The listing builds one solid part. Answer for the finished solid, in the listing's coordinates (mm). A direction names the side the tool comes from. Give positions to 0.01 mm unless a question says otherwise; leave off trailing zeros. Write each loop counter-clockwise with the first axis right and the second up, starting at its lowest first coordinate (ties: lowest second). Pieces come first, ordered by that corner, then holes.
```python
from build123d import *

# Parameters (mm, degrees)
SKETCH1_W           = 6.9
SKETCH1_H           = 6.9
BOSS_EXTRUDE1_DEPTH = 7.5
FILLET2_R           = 3.5
FILLET3_R           = 3.5
FILLET4_R           = 3.5
FILLET5_DEPTH       = 7.5
SKETCH2_R           = 3.429778851
BOSS_EXTRUDE3_DEPTH = 7.5
SKETCH4_W           = 6.879778851
SKETCH4_H           = 1.06
CUT_EXTRUDE6_DEPTH  = 15
CUT_EXTRUDE8_DEPTH  = 15


with BuildPart() as part:
    # Sketch1 → Boss-Extrude1 (new body)
    with BuildSketch(Plane.XY):
        with Locations((3.45, 3.45)):
            Rectangle(SKETCH1_W, SKETCH1_H)
        Polygon((3.45, 5.9), (4.4, 5.9), (4.4, 4.4), (5.9, 4.4), (5.9, 2.5), (4.4, 2.5), (4.4, 1), (2.5, 1), (2.5, 2.5), (1, 2.5), (1, 4.4), (2.5, 4.4), (2.5, 5.9), align=None, mode=Mode.SUBTRACT)
    extrude(amount=BOSS_EXTRUDE1_DEPTH)

    # Fillet2
    fillet2_edges = [part.edges().sort_by_distance(p)[0] for p in [
        (0, 6.9, 3.75),
    ]]
    fillet(fillet2_edges, radius=FILLET2_R)

    # Fillet3
    # the kernel refuses this fillet: 3.5 mm, written as the material it takes off along each edge
    with BuildSketch(Plane(origin=(6.9, 6.9, -8.746427842), x_dir=(-1, 0, 0), z_dir=(0, 0, 1))) as fillet3_piece_1:
        with BuildLine():
            CenterArc((3.5, 3.498571137), FILLET3_R, 180, 88.362754922)
            Line((0, 3.498571137), (-0.07, 3.498571137))
            Line((-0.07, 3.498571137), (-0.07, 0))
            Line((-0.07, 0), (0, -0.07))
            ThreePointArc((0, -0.07), (1.7, -0.07), (3.398, -0.069971423))
            Line((3.398, -0.069971423), (3.4, 0))
        make_face()
    extrude(amount=24.992855685, mode=Mode.SUBTRACT)

    # Fillet4
    # the kernel refuses this fillet: 3.5 mm, written as the material it takes off along each edge
    with BuildSketch(Plane(origin=(6.9, 0, -8.746529216), x_dir=(0, 1, 0), z_dir=(0, 0, 1))) as fillet4_piece_1:
        with BuildLine():
            CenterArc((3.5, 3.498611686), FILLET4_R, 180, 88.386155146)
            Line((0, 3.498611686), (-0.07, 3.498611686))
            Line((-0.07, 3.498611686), (-0.07, 0))
            Line((-0.07, 0), (0, -0.07))
            ThreePointArc((0, -0.07), (1.700714432, -0.07), (3.39945744, -0.069972234))
            Line((3.39945744, -0.069972234), (3.401428863, 0))
        make_face()
    extrude(amount=24.993058431, mode=Mode.SUBTRACT)

    # Fillet5: read off the stored shape, not the designer's step
    # Fillet5 outline → Fillet5 (cut)
    with BuildSketch(Plane.XY):
        with BuildLine():
            Line((0, 0), (3.401388314, 0))
            ThreePointArc((3.401388314, 0), (1.007751346, 1.041234576), (0.000347304, 3.449305272))
            ThreePointArc((0.000347304, 3.449305272), (8.6827e-05, 3.424653248), (0, 3.4))
            Line((0, 3.4), (0, 0))
        make_face()
    extrude(amount=FILLET5_DEPTH, mode=Mode.SUBTRACT)

    # Sketch2 → Boss-Extrude3 (add)
    with BuildSketch(Plane.XY):
        with Locations((3.45, 3.449305272)):
            Circle(SKETCH2_R)
        with BuildLine():
            Line((5.5103837, 5.418396181), (1.3896163, 5.418396181))
            ThreePointArc((1.3896163, 5.418396181), (0.6, 3.449305272), (1.3896163, 1.480214363))
            Line((1.3896163, 1.480214363), (5.5103837, 1.480214363))
            ThreePointArc((5.5103837, 1.480214363), (6.3, 3.449305272), (5.5103837, 5.418396181))
        make_face(mode=Mode.SUBTRACT)
    extrude(amount=-BOSS_EXTRUDE3_DEPTH)

    # Sketch4 → Cut-Extrude6 (cut)
    with BuildSketch(Plane(origin=(0, 0, -7.5), x_dir=(-1, 0, 0), z_dir=(0, 0, -1))):
        with Locations((-3.439889426, 0.53)):
            Rectangle(SKETCH4_W, SKETCH4_H)
    extrude(amount=-CUT_EXTRUDE6_DEPTH, mode=Mode.SUBTRACT)

    # Sketch6 → Cut-Extrude8 (cut)
    with BuildSketch(Plane(origin=(0, 0, -7.5), x_dir=(-1, 0, 0), z_dir=(0, 0, -1))):
        Polygon((-3.455260778, 6.975766387), (-6.044608069, 6.975766387), (-6.044608069, 5.876947105), (-3.455260778, 5.876947105), (-1.008353024, 5.876947105), (-1.008353024, 6.975766387), align=None)
    extrude(amount=-CUT_EXTRUDE8_DEPTH, mode=Mode.SUBTRACT)


solid = part.part
```
Item 1: Each of these flat-tipped pins is pushed along its axis until it touches: P1, Ø0.7, axis at y = 2, z = 4.5, coming from the +X side; P2, Ø1.5, axis at x = 5, y = 4.5, coming from the -Z side; P3, Ø1.2, axis at y = 5.5, z = 3, coming from the +X side. Where does it stop, or does it pass through?
Conclusion:
P1: stops at x = 6.71
P2: stops at z = 0
P3: stops at x = 6.56
Item 2: Which of the six approach directions +Z, -Z, +X, -X, +Y, -Y give full straight-line access (tool end or side, diameter ignored) to faces 4 (the face through (2.5, 5, 4)), 5 (the face through (6.3, 3.4, -3.7)), 6 (the face through (6.88, 3.44, -3.7)), 7 (the face through (0.27, 4.75, 3.8)), 8 (the face through (3.4, 5.6, -7.5))?
Conclusion:
face 4: +Z, +Y, -Y
face 5: -Z
face 6: -Z, +X
face 7: +Z, -Z, -X, +Y
face 8: -Z, +X, -X, +Y, -Y
Item 3: A cutting plane is placed at B-B, the plane x = 2.25. Give the vertices of the cut face in (y, z).
Conclusion:
outline: (1.06, -7.5) - (1.48, -7.5) - (1.48, 0) - (2.5, 0) - (2.5, 7.5) - (1.06, 7.5) - close; (4.4, 0) - (5.42, 0) - (5.42, -7.5) - (5.88, -7.5) - (5.88, 7.5) - (4.4, 7.5) - close
Item 4: A cutting plane is placed at A-A, the plane z = 3. Give the vertices of the cut face in (x, y).
Conclusion:
outline: (0, 3.45) arc R3.5 ccw to (0.99, 1.06) - (2.5, 1.06) - (2.5, 2.5) - (1, 2.5) - (1, 4.4) - (2.5, 4.4) - (2.5, 5.88) - (1.03, 5.88) arc R3.5 ccw to start; (4.4, 1.06) - (5.91, 1.06) arc R3.5 ccw to (6.9, 3.4) arc R3.5 ccw to (5.87, 5.88) - (4.4, 5.88) - (4.4, 4.4) - (5.9, 4.4) - (5.9, 2.5) - (4.4, 2.5) - close
Item 5: Determine the mould class of faces 1 (the face through (0.7, 3.5, 7.5)), 2 (the face through (0.273, 2.143, 3.698)), 3 (the face through (1, 3, 4)) for opening direction X: pulls with the +X half, pulls with the -X half, needs draft (parallel to the pull), parting line crosses it, or undercut.
Conclusion:
face 1: needs draft
face 2: pulls with the -X half
face 3: undercut
Item 6: Consider probe 1 along Y at (x, z) = (2.25, -2.75); probe 2 along Y at (x, z) = (2, 0.75); probe 3 along Z at (x, y) = (1.25, 4.85). Determine where each line is inside the solid, lowest interval first.
Conclusion:
probe 1: y = 1.06 to 1.48, 5.42 to 5.88
probe 2: y = 1.06 to 2.5, 4.4 to 5.88
probe 3: z = 0 to 7.5
Item 7: A cutting plane is placed at D-D, the plane z = -3. Give the vertices of the cut face in (x, y).
Conclusion:
outline: (0.99, 1.06) - (5.91, 1.06) arc R3.43 ccw to (5.87, 5.88) - (1.03, 5.88) arc R3.43 ccw to start; hole (1.39, 1.48) - (5.51, 1.48) arc R2.85 ccw to (5.51, 5.42) - (1.39, 5.42) arc R2.85 ccw to start
